Build history of the part. All positions in model axes, mm. A direction names the side the tool comes from. Round coordinates to 2 decimals unless told otherwise and drop trailing zeros. Loops run counter-clockwise (first coordinate to the right, second up) from the corner with the lowest first, then second, coordinate; pieces in that order, holes last. Notation, with made-up numbers: (29.5, 58) - (59.5, 58) arc R23 cw to (59.5, 96) - close; hole circle Ø11 at (-27.5, 5). An arc over 180 degrees is marked (long way). Use one line per item in the form item = value. Start each with the question number.
Q1. Mould opens along Y. For faces 1 (the face through (2.808, 4.437, 3.624)), 2 (the face through (4.561, 5.673, 1.208)), 3 (the face through (3, 0, 1)) say: released by +Y, released by -Y, zero draft, split by the parting line, or undercut.
Q2. Saw through at A-A (z = 0.6). Give the cut face in (x, y) (3 decimals).
Q3. Drill centre lines: line 1 (X direction, y = 3.5, z = 1.1); line 2 (X direction, y = 6, z = 2.65); line 3 (Z direction, x = 2.25, y = 8.5). Where is each one in solid material? Low to high.
Q4. Saw through at C-C (x = 1.2). Give the cut face in (y, z).
Q5. 3-axis set-ups, long thin cutter, end or side, ignore diameter. For faces 4 (the face through (3.13, 4.44, 5.09)), 5 (the face through (1, 5, 2)): which of +Z, -Z, +X, -X, +Y, -Y reach the whole face in a straight line?
Q6. Saw through at B-B (x = 1.8). Give the cut face in (y, z).
Q7. Saw through at D-D (y = 2.5). Give the cut face in (x, z) (3 decimals).
Q8. Pin check, flat tips, straight feed: pin 1 (3 mm diameter, centred on x = 1.5, y = 8, fed in from +Z); pin 2 (1.4 mm diameter, centred on x = 1, y = 5, fed in from -Z). Stop position of each tip, or through.
Autodesk Inventor part; units mm, degrees
ref_plane "screwMaxDist" through (2.575, 0, 2) normal (0, 0, 1) x (1, 0, 0)
ref_plane "YZ Plane" through (0, 0, 0) normal (1, 0, 0) x (0, 1, 0)
ref_plane "XZ Plane" through (0, 0, 0) normal (0, 1, 0) x (-1, 0, 0)
sketch "Sketch1" plane through (0, 0, 0) normal (0, 1, 0) x (-1, 0, 0)
  circle A0 centre (-2.575, 2.575) radius 1.075
  circle A1 centre (-2.575, 2.575) radius 2.575
  line L0 (0, 0) -> (-7.3028, 0) construction
  line L1 (0, 0) -> (0, 4.3038) construction
  dimension "d0" = 2.15
  dimension "d1" = 5.15
extrude "Extrusion1" add sketch "Sketch1" along normal blind 9
ref_plane "Work Plane1" through (2.575, 0, 1.5) normal (0, 0, 1) x (1, 0, 0)
ref_plane "screwMaxDist" through (2.575, 0, 2) normal (0, 0, 1) x (1, 0, 0)
sketch "Sketch2" plane through (0, 0, 0) normal (0, 0, 1) x (1, 0, 0)
  line L0 (5.15, 9) -> (0, 9)
  circle A0 centre (2.575, 4.85) radius 2.15
  line L1 (5.15, 9) -> (0, 9)
  line L2 (5.15, 0) -> (0, 0)
  line L3 (0, 0) -> (0, 9)
  line L4 (0, 7) -> (5.15, 7)
  line L5 (5.15, 0) -> (5.15, 9)
  dimension "d5" = 4.3
  dimension "d15" = 2
  dimension "d16" = 2.575
  dimension "d17" = 2.575
extrude "Extrusion2" cut sketch "Sketch2" along normal up to surface (2 mm away) contours A0
equation "\"d16\" = d17"
properties part number "motor_shaft_adapter" material "ABS Plastic"
Report:
q1.face_1 = zero draft
q1.face_2 = undercut
q1.face_3 = released by -Y
q2.outline = (0.923, 0) - (4.227, 0) - (4.227, 3.474) arc R2.15 cw to (0.923, 3.474) - close; (0.923, 6.226) arc R2.15 cw to (4.227, 6.226) - (4.227, 9) - (0.923, 9) - close
q3.line_1 = 0.46 to 0.9, 4.25 to 4.69
q3.line_2 = 0 to 1.5, 3.65 to 5.15
q3.line_3 = 0.02 to 1.55, 3.6 to 5.13
q4.outline = (0, 0.4) - (3.2, 0.4) - (3.2, 2) - (6.5, 2) - (6.5, 0.4) - (9, 0.4) - (9, 4.75) - (0, 4.75) - close
q5.face_4 = +Y, -Y
q5.face_5 = -Z
q6.outline = (0, 0.12) - (2.84, 0.12) - (2.84, 1.83) - (0, 1.83) - close; (0, 3.32) - (9, 3.32) - (9, 5.03) - (0, 5.03) - close; (6.86, 0.12) - (9, 0.12) - (9, 1.83) - (6.86, 1.83) - close
q7.outline = circle Ø5.15 at (2.575, 2.575); hole circle Ø2.15 at (2.575, 2.575)
q8.pin_1 = 5.15
q8.pin_2 = 1.01
